Can you work these out from the model? Positions are in its coordinate system, mm. Face numbers are marked on the shaded views. A direction names the side the tool comes from. Round coordinates to 2 decimals unless told otherwise and drop trailing zeros. Write each loop counter-clockwise with the first axis right and the second up, starting at its lowest first coordinate (ties: lowest second). Pieces come first, ordered by that corner, then holes.
Q1. For the marked faces 1 and 2, which set-ups out of +Z, -Z, +X, -X, +Y, -Y let a thin tool reach every point of the face, with its end or its side?
Q2. I'm going to push flat-ended pins straight in: pin 1 Ø10 at (y, z) = (-18.5, -7.5) entering from +X; pin 2 Ø4.5 at (x, z) = (3, 3.5) entering from +Y. Where does each tip first touch, or does it pass through?
Q3. If we section it at A-A (z = 0): Please give me the cut outline in (x, y), plus the area to 3 significant figures.
Q4. If we section it at C-C (y = 7): Please give me the cut outline in (x, z) (3 decimals), plus the area to 3 significant figures.
Q5. If we section it at B-B (x = 20.5): Please give me the cut outline in (y, z) (3 decimals).
Q6. Please list where these lines run through material, in increasing order: line 1 along X through (y, z) = (7, 2); line 2 along X through (y, z) = (20, -7.75).
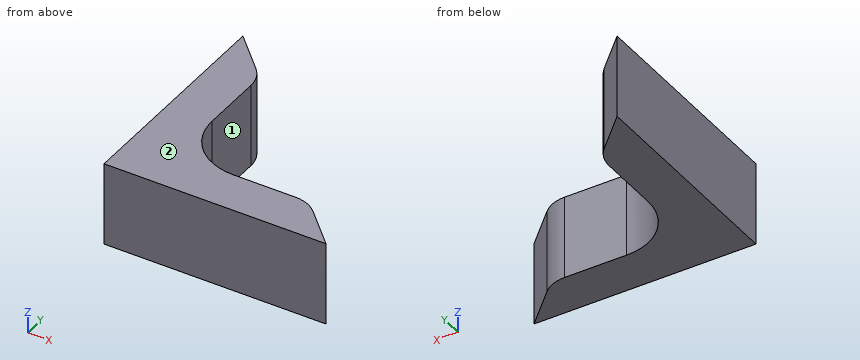
from build123d import *

# Parameters (mm, degrees)
F1_DEPTH = 9.525
F2_R     = 13.061378
F3_R     = 7.62


with BuildPart() as f1:
    # F0 (on Top) → F1 (new body, symmetric)
    with BuildSketch(Plane.XY):
        Polygon((-25.4, -25.4), (25.4, -25.4), (15.24, -15.24), (-15.24, -15.24), (-15.24, 15.24), (-25.4, 25.4), align=None)
    extrude(amount=F1_DEPTH, both=True)

    # F2
    f2_edges = [f1.edges().sort_by_distance(p)[0] for p in [
        (-15.24, -15.24, 0),
    ]]
    fillet(f2_edges, radius=F2_R)

    # F3
    f3_edges = [f1.edges().sort_by_distance(p)[0] for p in [
        (-15.24, 15.24, 0),
        (15.24, -15.24, 0),
    ]]
    fillet(f3_edges, radius=F3_R)


solid = f1.part
A:
1. face 1: +Z, -Z, +X, +Y
1. face 2: +Z, +X, -X, +Y, -Y
2. pin 1: stops at x = 23.5
2. pin 2: stops at y = -15.24
3. outline: (-25.4, -25.4) - (25.4, -25.4) - (17.47, -17.47) arc R7.62 ccw to (12.08, -15.24) - (-2.18, -15.24) arc R13.06 cw to (-15.24, -2.18) - (-15.24, 12.08) arc R7.62 ccw to (-17.47, 17.47) - (-25.4, 25.4) - close
3. area: 860 mm2
4. outline: (-25.4, -9.525) - (-15.24, -9.525) - (-15.24, 9.525) - (-25.4, 9.525) - close
4. area: 194 mm2
5. outline: (-25.4, -9.525) - (-20.5, -9.525) - (-20.5, 9.525) - (-25.4, 9.525) - close
6. line 1: x = -25.4 to -15.24
6. line 2: x = -25.4 to -20
